Read the model definition and answer for the solid it produces. Units are mm, in the model's axes. A direction names the side the tool comes from. Coordinates: 2 decimals unless noted, no trailing zeros. Write each loop counter-clockwise with the first axis right and the second up, starting at its lowest first coordinate (ties: lowest second). Pieces come first, ordered by that corner, then holes.
Item 1: Each of these flat-tipped pins is pushed along its axis until it touches: P1, Ø4, axis at y = -12.5, z = -11, coming from the +X side; P2, Ø10.5, axis at x = 0, y = 15, coming from the -Z side; P3, Ø5.5, axis at y = 5.5, z = -31.5, coming from the -X side. Where does it stop, or does it pass through?
Item 2: A tool of negligible diameter and unlimited length cuts with its end or side. For faces 1 (the face through (-2, 0, 23.349)), 2 (the face through (15, 7, -32)), 3 (the face through (-0.27, 2.28, -27.36)), 4 (the face through (1.4, -1.4, 25.349)), from which of +Z, -Z, +X, -X, +Y, -Y can it reach the whole face along a straight path? Write none if from no direction.
Item 3: Section D-D (y = 9.5) is taken. Give the vertices of the cut face in (x, z).
Item 4: Section B-B (x = 20.5) is taken. Give the vertices of the cut face in (y, z), then the cut area to 3 significant figures.
Item 5: Section C-C (z = 0.5) is taken. Give the vertices of the cut face in (x, y).
Item 6: Determine the mould class of faces 5 (the face through (1.4, -16.4, 25.349)), 6 (the face through (-15, 7, -32)), 7 (the face through (-8.859, -12.297, -36.321)) for opening direction Y: released by +Y, released by -Y, zero draft, split by the parting line, or undercut.
Item 7: Section A-A (y = -6.5) is taken. Give the vertices of the cut face in (x, z), then the cut area to 3 significant figures.
Item 8: Straight lines are drawn through the part: probe 1 along Y at (x, z) = (0, -26.75); probe 2 along Y at (x, z) = (0, 26.2); probe 3 along Y at (x, z) = (0, 23.9). For each, find the intervals that lie inside material, in ascending order.
from build123d import *

# Parameters (mm, degrees)
BOSS_EXTRUDE1_DEPTH            = 22.5
CUT_EXTRUDE1_DEPTH             = 36
CBORE_FOR_M3_SHCS1_D           = 3.4
CBORE_FOR_M3_SHCS1_DEPTH       = 5
CBORE_FOR_M3_SHCS1_CBORE_D     = 6.5
CBORE_FOR_M3_SHCS1_CBORE_DEPTH = 3
CBORE_FOR_M3_SHCS1_TIP         = 1.021463052
M3X0_5_TAPPED_HOLE1_D          = 2.5
M3X0_5_TAPPED_HOLE1_DEPTH      = 27.571916674
M3X0_5_TAPPED_HOLE1_TIP        = 0.751075774
FILLET2_R                      = 4
TOLERANCING_START              = -22.5
TOLERANCING_DEPTH              = 45


# Read off the part's stored shape, not the designer's step: Tolerancing
with BuildPart() as part:
    # Sketch1 → Boss-Extrude1 (new, symmetric)
    with BuildSketch(Plane(origin=(0, 0, 0), x_dir=(1, 0, 0), z_dir=(0, 1, 0))):
        with BuildLine():
            Line((-15, -28.348661632), (15, -28.348661632))
            ThreePointArc((15, -28.348661632), (36.566832412, 5), (15, 38.348661632))
            Line((15, 38.348661632), (-15, 38.348661632))
            ThreePointArc((-15, 38.348661632), (-36.566832412, 5), (-15, -28.348661632))
        make_face()
        with BuildLine():
            Line((-10, -23.348661632), (10, -23.348661632))
            ThreePointArc((10, -23.348661632), (0, 25.4), (-10, -23.348661632))
        make_face(mode=Mode.SUBTRACT)
    extrude(amount=BOSS_EXTRUDE1_DEPTH, both=True)

    # Sketch4 → Cut-Extrude1 (cut)
    with BuildSketch(Plane(origin=(0, 22.5, 0), x_dir=(1, 0, 0), z_dir=(0, 1, 0))):
        Polygon((-10, 38.348661632), (-10, 34.348661632), (-15, 34.348661632), (-15, 29.348661632), (15, 29.348661632), (15, 34.348661632), (10, 34.348661632), (10, 38.348661632), align=None)
    extrude(amount=-CUT_EXTRUDE1_DEPTH, mode=Mode.SUBTRACT)

    # CBORE for M3 SHCS1
    with Locations(Plane.XY.offset(28.348661632)):
        with Locations((0, 0), (0, 15), (0, -15)):
            CounterBoreHole(CBORE_FOR_M3_SHCS1_D / 2, CBORE_FOR_M3_SHCS1_CBORE_D / 2, CBORE_FOR_M3_SHCS1_CBORE_DEPTH, depth=CBORE_FOR_M3_SHCS1_DEPTH)
            with Locations((0, 0, -(CBORE_FOR_M3_SHCS1_DEPTH + CBORE_FOR_M3_SHCS1_TIP / 2))):  # 118° drill point
                Cone(0, CBORE_FOR_M3_SHCS1_D / 2, CBORE_FOR_M3_SHCS1_TIP, mode=Mode.SUBTRACT)

    # M3x0.5 Tapped Hole1
    with Locations(Plane(origin=(0, 0, -29.348661632), x_dir=(-1, 0, 0), z_dir=(0, 0, -1))):
        with Locations((0, 3.5), (0, -6.5)):
            Hole(M3X0_5_TAPPED_HOLE1_D / 2, depth=M3X0_5_TAPPED_HOLE1_DEPTH)
            with Locations((0, 0, -(M3X0_5_TAPPED_HOLE1_DEPTH + M3X0_5_TAPPED_HOLE1_TIP / 2))):  # 118° drill point
                Cone(0, M3X0_5_TAPPED_HOLE1_D / 2, M3X0_5_TAPPED_HOLE1_TIP, mode=Mode.SUBTRACT)

    # Fillet2
    fillet2_edges = [part.edges().sort_by_distance(p)[0] for p in [
        (10, -13.5, -36.348661632),
        (15, -13.5, -31.848661632),
        (-15, -13.5, -31.848661632),
        (-10, -13.5, -36.348661632),
    ]]
    fillet(fillet2_edges, radius=FILLET2_R)

    # Tolerancing outline → Tolerancing (cut)
    with BuildSketch(Plane(origin=(0, 0, 0), x_dir=(1, 0, 0), z_dir=(0, 1, 0)).offset(TOLERANCING_START)):
        with BuildLine():
            ThreePointArc((10.126327074, -23.348661632), (0, 25.45), (-10.126327074, -23.348661632))
            Line((-10.126327074, -23.348661632), (-10, -23.348661632))
            ThreePointArc((-10, -23.348661632), (0, 25.4), (10, -23.348661632))
            Line((10, -23.348661632), (10.126327074, -23.348661632))
        make_face()
    extrude(amount=TOLERANCING_DEPTH, mode=Mode.SUBTRACT)


solid = part.part
Established:
1. P1: stops at x = 36.35
1. P2: stops at z = -29.35
1. P3: stops at x = -27.8
2. face 1: +Y, -Y
2. face 2: +Y
2. face 3: -Z
2. face 4: +Z
3. outline: (-15, -38.35) - (-10, -38.35) - (-10, -34.35) - (-15, -34.35) - (-15, -29.35) - (15, -29.35) - (15, -34.35) - (10, -34.35) - (10, -38.35) - (15, -38.35) arc R36.57 ccw to (15, 28.35) - (-15, 28.35) arc R36.57 ccw to start; hole (-10.13, 23.35) arc R25.45 ccw (long way) to (10.13, 23.35) - close
4. outline: (-22.5, -35.28) - (22.5, -35.28) - (22.5, -15.08) - (-22.5, -15.08) - close; (-22.5, 15.08) - (22.5, 15.08) - (22.5, 25.28) - (-22.5, 25.28) - close
4. area: 1,370 mm2
5. outline: (-36.15, -22.5) - (-25.45, -22.5) - (-25.45, 22.5) - (-36.15, 22.5) - close; (25.45, -22.5) - (36.15, -22.5) - (36.15, 22.5) - (25.45, 22.5) - close
6. face 5: undercut
6. face 6: zero draft
6. face 7: released by +Y
7. outline: (-15, -38.35) - (-10, -38.35) - (-10, -34.35) - (-15, -34.35) - (-15, -29.35) - (-1.25, -29.35) - (-1.25, -25.42) arc R25.45 cw to (-10.13, 23.35) - (10.13, 23.35) arc R25.45 cw to (1.25, -25.42) - (1.25, -29.35) - (15, -29.35) - (15, -34.35) - (10, -34.35) - (10, -38.35) - (15, -38.35) arc R36.57 ccw to (15, 28.35) - (-15, 28.35) arc R36.57 ccw to start
7. area: 1,820 mm2
8. probe 1: y = -22.5 to -7.75, -5.25 to 2.25, 4.75 to 22.5
8. probe 2: y = -22.5 to -18.25, -11.75 to -3.25, 3.25 to 11.75, 18.25 to 22.5
8. probe 3: y = -22.5 to -16.7, -13.3 to -1.7, 1.7 to 13.3, 16.7 to 22.5
